Autodesk Inventor part; units mm, degrees
ref_plane "YZ Plane" through (0, 0, 0) normal (1, 0, 0) x (0, 1, 0)
ref_plane "XZ Plane" through (0, 0, 0) normal (0, 1, 0) x (-1, 0, 0)
ref_plane "XY Plane" through (0, 0, 0) normal (0, 0, 1) x (1, 0, 0)
sketch "Sketch2" plane through (0, 0, 0) normal (0, 0, 1) x (1, 0, 0)
  circle A0 centre (0, 0) radius 1.5
  dimension "Diameter" = 3
extrude "Extrusion1" add sketch "Sketch2" against normal blind 4.14
sketch "Sketch3" plane through (0, 0, 0) normal (0, 0, 1) x (1, 0, 0)
  circle A0 centre (0, 0) radius 1.5
extrude "Extrusion2" add sketch "Sketch3" along normal blind 1.86 draft 45
sketch "Sketch4" plane through (0, 0, 1.86) normal (0, 0, 1) x (1, 0, 0)
  circle A0 centre (0, 0) radius 3.36
  line L0 (0.5774, 1) -> (1.1547, 0)
  line L1 (1.1547, 0) -> (0.5774, -1)
  line L2 (0.5774, -1) -> (-0.5774, -1)
  line L3 (-0.5774, -1) -> (-1.1547, 0)
  line L4 (-1.1547, 0) -> (-0.5774, 1)
  line L5 (-0.5774, 1) -> (0.5774, 1)
  line L6 (0, 0) -> (1.1547, 0) construction
  dimension "Hex_Width" = 2
extrude "Extrusion3" cut sketch "Sketch4" against normal blind 1.1 contours L0 L1 L2 L3 L4 L5
thread "Thread1"
chamfer "Chamfer1" distance 0.3 angle 45 1 edges at (-1.5, 0, -4.14)
fillet "Fillet1" radius 0.1 1 edges at (-3.36, 0, 1.86)
equation "\"Length1\" = Length - Head_Height"
equation "\"Thread_Length\" = Length1"
equation "\"Length\" = 6"
properties part number "SCREW,FLAT-HD,SS,18-8,M03X0_50X006MM" material "Steel, 1018, CRS"
Geometry check sheet. Reference: the model listing, model coordinates, mm. A direction names the side the tool comes from. Coordinates: 2 decimals unless noted, no trailing zeros. Order: outer loops, then holes, each group sorted by start corner. A loop starts at its lowest first (then second) coordinate and runs counter-clockwise, first axis right, second up. Notation, with made-up numbers: (33, 3) - (52, 3) arc R15 ccw to (52, 16) - close; hole circle Ø6 at (-24.75, 9). An arc over 180 degrees is marked (long way). Answer in a Markdown table with one row per item. Add a question column.
1) Cross-section at A-A, the plane z = 1.5. Record the cut outline in (x, y), then the cut area to 3 significant figures.
2) Cross-section at C-C, the plane z = -2.5. Record the cut outline in (x, y), then the cut area to 3 significant figures.
3) Release check for a two-part mould opening along Y. For faces 4 (the conical face through (-0.35, -1.57, 0.11)), 5 (the flat face through (0, 0, -4.14)), 6 (the flat face through (-0.87, 0.49, 1.32)) record: +Y half, -Y half, draft (parallel to the pull), parting line (faces both ways), or undercut.
4) Gauge pin test, flat ends, axial feed: P1, Ø2, axis at x = -0.5, y = 0, coming from the +Z side; P2, Ø3, axis at x = -2.5, z = 0.5, coming from the -Y side; P3, Ø1.2, axis at x = 0, z = 1, coming from the +Y side; P4, Ø2, axis at y = 0, z = -2.5, coming from the +X side. Record the tip position at first contact, or that the pin passes through.
5) Cross-section at B-B, the plane x = 0. Record the cut outline in (y, z), then the cut area to 3 significant figures.
6) Set-up check for faces 1 (the flat face through (-1, 1, 1.86)), 2 (the cylindrical face through (-1.5, 0.07, -1.89)), 3 (the flat face through (-0.86, -0.51, 1.32)): record each of +Z, -Z, +X, -X, +Y, -Y from which the full face is reachable in a straight line by a thin tool's end or side.
7) Material ranges on line 1 along Z through (x, y) = (-0.75, 0); line 2 along Z through (x, y) = (2.5, 0); line 3 along Y through (x, z) = (-1, 1.5), recorded low to high. Write a range as [from, to].
Check result:
| question | item | result |
|---|---|---|
| 1 | outline | circle Ø6 at (0, 0); hole (-1.15, 0) - (-0.58, -1) - (0.58, -1) - (1.15, 0) - (0.58, 1) - (-0.58, 1) - close |
| 1 | area | 24.8 mm² |
| 2 | outline | circle Ø3 at (0, 0) |
| 2 | area | 7.07 mm² |
| 3 | face 4 | parting line |
| 3 | face 5 | draft |
| 3 | face 6 | undercut |
| 4 | P1 | stops at z = 1.86 |
| 4 | P2 | stops at y = -2.77 |
| 4 | P3 | stops at y = 3.1 |
| 4 | P4 | stops at x = 1.5 |
| 5 | outline | (-3.19, 1.69) - (-1.5, 0) - (-1.5, -3.84) - (-1.2, -4.14) - (1.2, -4.14) - (1.5, -3.84) - (1.5, 0) - (3.19, 1.69) arc R0.1 ccw to (3.12, 1.86) - (1, 1.86) - (1, 0.76) - (-1, 0.76) - (-1, 1.86) - (-3.12, 1.86) arc R0.1 ccw to start |
| 5 | area | 19.1 mm² |
| 6 | face 1 | +Z, +X, -X, +Y, -Y |
| 6 | face 2 | -Z |
| 6 | face 3 | +Z |
| 7 | line 1 | z = [-4.14, 0.76] |
| 7 | line 2 | z = [1, 1.86] |
| 7 | line 3 | y = [-2.83, -0.27], [0.27, 2.83] |
